from build123d import *

# Parameters (mm, degrees)
F1_DEPTH = 63.5
F0_W     = 25.4827047348
F0_H     = 19.05
F2_DEPTH = 25.4
F3_DEPTH = 7.9375
F5_R     = 6.35
F6_R     = 6.35


with BuildPart() as f1:
    # F0 (on Front) → F1 (new body, symmetric)
    with BuildSketch(Plane.XZ):
        Polygon((41.275, -9.525), (41.275, 9.525), (22.225, 9.525), (-41.275, 9.525), (-41.275, -9.525), align=None)
    extrude(amount=F1_DEPTH, both=True)

    # F0 (on Front) → F2 (join, symmetric)
    with BuildSketch(Plane.XZ):
        with BuildLine():
            Line((22.225, 9.525), (41.275, 9.525))
            Line((41.275, 9.525), (41.275, 27.0061871217))
            ThreePointArc((41.275, 27.0061871217), (45.7715909854, 38.0763015427), (56.7140467144, 42.8752))
            Line((56.7140467144, 42.8752), (60.2422952652, 42.8752))
            Line((60.2422952652, 42.8752), (60.2422952652, 61.9252))
            Line((60.2422952652, 61.9252), (56.5033435204, 61.9252))
            ThreePointArc((56.5033435204, 61.9252), (32.2267166835, 51.4721956585), (22.225, 27.0061871217))
            Line((22.225, 27.0061871217), (22.225, 9.525))
        make_face()
        with Locations((72.9836476326, 52.4002)):
            Rectangle(F0_W, F0_H)
    extrude(amount=F2_DEPTH, both=True)

    # F0 (on Front) → F3 (join, symmetric)
    with BuildSketch(Plane.XZ):
        with BuildLine():
            Line((-41.275, 9.525), (22.225, 9.525))
            Line((22.225, 9.525), (22.225, 27.0061871217))
            ThreePointArc((22.225, 27.0061871217), (32.2267166835, 51.4721956585), (56.5033435204, 61.9252))
            Line((56.5033435204, 61.9252), (60.2422952652, 61.9252))
            Line((60.2422952652, 61.9252), (60.2422952652, 62.2294992208))
            Line((60.2422952652, 62.2294992208), (56.5033435204, 62.2294992208))
            add(Edge.make_bspline(
                [(-41.275, 9.525), (-3.9314110763, 49.0912124515), (24.1732224822, 58.5743710399), (56.5033435204, 62.2294992208)],
                knots=[0, 0, 0, 0, 111.0782098331, 111.0782098331, 111.0782098331, 111.0782098331], degree=3))
        make_face()
    extrude(amount=F3_DEPTH, both=True)

    # F0 (on Front) → F4 (revolve)
    with BuildSketch(Plane.XZ):
        Polygon((85.725, 61.9252), (85.725, 42.8752), (85.725, 38.1), (111.0422952652, 38.1), (111.0422952652, 66.675), (85.725, 66.675), (85.725, 62.2294992208), align=None)
    revolve(axis=Axis((85.725, 0, 52.5523496104), (0, 0, -1)))

    # F5
    f5_edges = [f1.edges().sort_by_distance(p)[0] for p in [
        (41.275, -63.5, 0),
        (41.275, 63.5, 0),
    ]]
    fillet(f5_edges, radius=F5_R)

    # F6
    f6_edges = [f1.edges().sort_by_distance(p)[0] for p in [
        (-41.275, -63.5, 0),
        (-41.275, 63.5, 0),
    ]]
    fillet(f6_edges, radius=F6_R)


solid = f1.part
Here's how the part is built. I have some questions about the finished solid (model axes, mm). A direction names the side the tool comes from. Give positions to 0.01 mm unless a question says otherwise; leave off trailing zeros. Order: outer loops, then holes, each group sorted by start corner. A loop starts at its lowest first (then second) coordinate and runs counter-clockwise, first axis right, second up. Notation, with made-up numbers: (42.25, 17) -> (46.25, 17) arc R7 cw to (46.25, 21) -> close; hole circle Ø10 at (55.25, -40). An arc over 180 degrees is marked (long way). Use a Markdown table: item, result. Add a question column.
Item 1: Imagine slicing it at D-D on x = 94. Please give me the cut outline in (y, z) (3 decimals), plus the area to 3 significant figures.
Item 2: Imagine slicing it at C-C on y = 38. Please give me the cut outline in (x, z) (3 decimals), plus the area to 3 significant figures.
Item 3: If we mould it in two halves opening along X, with no side actions, what happens to faces 1 (the face through (1, -36, 9.525)), 2 (the face through (60, -4, 42.875)), 3 (the face through (22.225, 17, 18))? For each: pulls with the +X half, pulls with the -X half, needs draft (parallel to the pull), parting line crosses it, or undercut.
Item 4: Imagine slicing it at A-A on x = 72.5. Please give me the cut outline in (y, z) (3 decimals).
Item 5: Imagine slicing it at B-B on y = 17. Please give me the cut outline in (x, z) (3 decimals).
Item 6: I need wall thicknesses on line 1 (Z direction, x = 26, y = 28) (3 decimals); line 2 (X direction, y = 39.5, z = -4.5) (3 decimals); line 3 (Y direction, x = 40, z = 58). Which ranges of each line are inside material? Lowest first, please.
Item 7: Will these pins go through, and if not, where does the flat tip stop? pin 1 (1.1 mm diameter, centred on x = 59, y = 1.5, fed in from +Z); pin 2 (1.5 mm diameter, centred on x = 76, z = 45, fed in from -Y); pin 3 (4 mm diameter, centred on x = 31, y = 32.5, fed in from +Z) (3 decimals).
Item 8: For faces 4 (the face through (58, 0, 62.229)), 5 (the face through (46, -25.4, 42)), 6 (the face through (9, 7.938, 30)), 7 (the face through (22.225, -17, 18)), 8 (the face through (45.7, -0.4, 38)), which set-ups out of +Z, -Z, +X, -X, +Y, -Y let a thin tool reach every point of the face, with its end or its side?
Data:
| question | item | result |
|---|---|---|
| 1 | outline | (-23.927, 38.1) -> (23.927, 38.1) -> (23.927, 66.675) -> (-23.927, 66.675) -> close |
| 1 | area | 1,370 mm² |
| 2 | outline | (-41.275, -9.525) -> (41.275, -9.525) -> (41.275, 9.525) -> (-41.275, 9.525) -> close |
| 2 | area | 1,570 mm² |
| 3 | face 1 | needs draft |
| 3 | face 2 | undercut |
| 3 | face 3 | pulls with the -X half |
| 4 | outline | (-25.4, 42.875) -> (-21.589, 42.875) -> (-21.589, 38.1) -> (21.589, 38.1) -> (21.589, 42.875) -> (25.4, 42.875) -> (25.4, 61.925) -> (21.589, 61.925) -> (21.589, 66.675) -> (-21.589, 66.675) -> (-21.589, 61.925) -> (-25.4, 61.925) -> close |
| 5 | outline | (-41.275, -9.525) -> (41.275, -9.525) -> (41.275, 27.006) arc R15.875 cw to (56.714, 42.875) -> (66.964, 42.875) -> (66.964, 38.1) -> (104.486, 38.1) -> (104.486, 66.675) -> (66.964, 66.675) -> (66.964, 61.925) -> (56.503, 61.925) arc R34.925 ccw to (22.225, 27.006) -> (22.225, 9.525) -> (-41.275, 9.525) -> close |
| 6 | line 1 | z = -9.525 to 9.525 |
| 6 | line 2 | x = -41.275 to 41.275 |
| 6 | line 3 | y = -7.94 to 7.94 |
| 7 | pin 1 | stops at z = 62.23 |
| 7 | pin 2 | stops at y = -25.4 |
| 7 | pin 3 | stops at z = 9.525 |
| 8 | face 4 | +Z, -X, +Y, -Y |
| 8 | face 5 | +Z, +X, -X, -Y |
| 8 | face 6 | +Z, -X, +Y |
| 8 | face 7 | +Z, -X, -Y |
| 8 | face 8 | -Z, +Y, -Y |
